Verification items for the finished model (mm, model axes). A direction names the side the tool comes from. Round coordinates to 2 decimals unless told otherwise and drop trailing zeros. Order: outer loops, then holes, each group sorted by start corner. A loop starts at its lowest first (then second) coordinate and runs counter-clockwise, first axis right, second up. Notation, with made-up numbers: (17.5, 31.5) -> (58.5, 31.5) arc R27 cw to (58.5, 47.5) -> close; hole circle Ø7 at (-31.75, -35). An arc over 180 degrees is marked (long way). Put each result on its own line as item: value.
from build123d import *

# Parameters (mm, degrees)
SKETCH1_R           = 12.7
BOSS_EXTRUDE1_DEPTH = 63.5
CUT_EXTRUDE1_DEPTH  = 25.4


with BuildPart() as part:
    # Sketch1 → Boss-Extrude1 (new body)
    with BuildSketch(Plane(origin=(0, 0, 0), x_dir=(1, 0, 0), z_dir=(0, 1, 0))):
        with Locations(Location((0, 0, 0), (0, 0, 270))):
            Circle(SKETCH1_R)
    extrude(amount=BOSS_EXTRUDE1_DEPTH)

    # Sketch2 → Cut-Extrude1 (cut)
    with BuildSketch(Plane.XZ):
        with BuildLine():
            Line((-10.16, 7.62), (-10.16, -7.62))
            ThreePointArc((-10.16, -7.62), (-12.7, 0), (-10.16, 7.62))
        make_face()
        with BuildLine():
            Line((10.16, 7.62), (10.16, -7.62))
            ThreePointArc((10.16, -7.62), (12.7, 0), (10.16, 7.62))
        make_face()
    extrude(amount=-CUT_EXTRUDE1_DEPTH, mode=Mode.SUBTRACT)

    # Sketch4 → 1/8 NPT Tapped Hole1 (revolve, cut)
    with BuildSketch(Plane(origin=(-10.16, 12.7, 0), x_dir=(0, 0, 1), z_dir=(0, 1, 0))):
        Polygon((0, 0), (0, 14.217468714), (4.2164, 11.684), (4.2164, 6.858), (4.936181096, 6.858), (5.1415188, 0), align=None)
    f_1_8_npt_tapped_hole1 = revolve(axis=Axis((-16.51, 12.7, 0), (1, 0, 0)), mode=Mode.SUBTRACT)

    # Mirror1: 1/8 NPT Tapped Hole1 across plane
    add(f_1_8_npt_tapped_hole1.mirror(Plane(origin=(0, 0, 0), x_dir=(0, 0, 1), z_dir=(1, 0, 0))), mode=Mode.SUBTRACT)


solid = part.part
Item 1: Material ranges on L1, parallel to Y at x = -1.5, z = 0; L2, parallel to X at y = 3, z = 6.5; L3, parallel to Y at x = -1, z = 1.75, recorded low to high. Write a range as [from, to].
Check sheet entries:
L1: y = [0, 8.48], [16.92, 63.5]
L2: x = [-10.16, 10.16]
L3: y = [0, 8.86], [16.54, 63.5]
Item 2: Section check D-D on y = 52.5. Record the boundary of the cut face in (x, z).
Check sheet entries:
outline: circle Ø25.4 at (0, 0)
Item 3: Section check B-B on y = 12.7. Record the boundary of the cut face in (x, z).
Check sheet entries:
outline: (-10.16, -7.62) arc R12.7 ccw to (10.16, -7.62) -> (10.16, -5.14) -> (3.3, -4.94) -> (3.3, -4.22) -> (-3.3, -4.22) -> (-3.3, -4.94) -> (-10.16, -5.14) -> close; (-10.16, 5.14) -> (-3.3, 4.94) -> (-3.3, 4.22) -> (3.3, 4.22) -> (3.3, 4.94) -> (10.16, 5.14) -> (10.16, 7.62) arc R12.7 ccw to (-10.16, 7.62) -> close
Item 4: Section check C-C on x = 0. Record the boundary of the cut face in (y, z), then the cut area to 3 significant figures.
Check sheet entries:
outline: (0, -12.7) -> (63.5, -12.7) -> (63.5, 12.7) -> (0, 12.7) -> close; hole circle Ø8.43 at (12.7, 0)
area: 1,560 mm^2
Item 5: Gauge pin test, flat ends, axial feed: pin 1 Ø6 at (x, y) = (-8.5, 37) entering from +Z; pin 2 Ø2 at (x, z) = (11.5, -2.5) entering from -Y; pin 3 Ø4 at (x, y) = (-4.5, 38) entering from -Z. Record the tip position at first contact, or that the pin passes through.
Check sheet entries:
pin 1: stops at z = 11.45
pin 2: stops at y = 25.4
pin 3: stops at z = -12.45
Item 6: Tool access check on faces 1 (the flat face through (3.302, 17, -1)), 2 (the flat face through (-11, 25.4, 0)), 3 (the flat face through (11, 25.4, 0)), 4 (the flat face through (0, 0, 0)), 5 (the flat face through (-3.302, 17, -1)). Record the directions out of +Z, -Z, +X, -X, +Y, -Y that give a thin tool (end or side, any length) a straight path to the whole face; none if there is none.
Check sheet entries:
face 1: +X
face 2: +Z, -Z, -X, -Y
face 3: +Z, -Z, +X, -Y
face 4: +Z, -Z, +X, -X, -Y
face 5: -X
Item 7: Section check A-A on z = 0. Record the boundary of the cut face in (x, y).
Check sheet entries:
outline: (-12.7, 25.4) -> (-10.16, 25.4) -> (-10.16, 17.84) -> (-3.3, 17.64) -> (-3.3, 16.92) -> (3.3, 16.92) -> (3.3, 17.64) -> (10.16, 17.84) -> (10.16, 25.4) -> (12.7, 25.4) -> (12.7, 63.5) -> (-12.7, 63.5) -> close; (-10.16, 0) -> (10.16, 0) -> (10.16, 7.56) -> (3.3, 7.76) -> (3.3, 8.48) -> (-3.3, 8.48) -> (-3.3, 7.76) -> (-10.16, 7.56) -> close
Item 8: Release check for a two-part mould opening along Z. For faces 6 (the conical face through (-6.78, 17.62, -1.09)), 7 (the cylindrical face through (0.558, 38.361, -12.688)), 8 (the flat face through (-10.16, 7, 0)), 9 (the cylindrical face through (0.05, 8.52, -0.55)) record: +Z half, -Z half, draft (parallel to the pull), parting line (faces both ways), or undercut.
Check sheet entries:
face 6: undercut
face 7: parting line
face 8: draft
face 9: undercut
